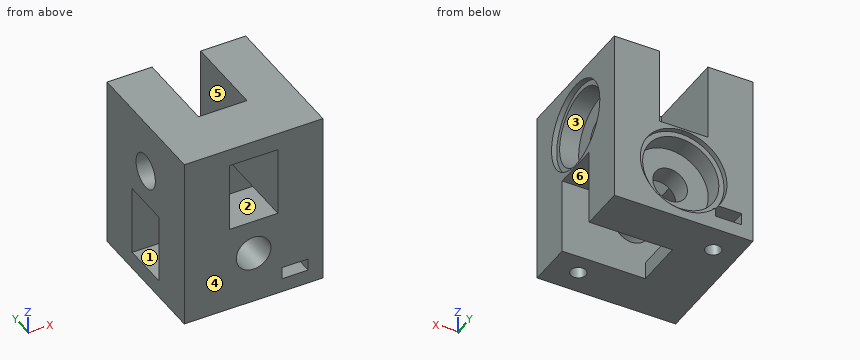
```python
from build123d import *

# Parameters (mm, degrees)
ESQUISSE1_W              = 40
ESQUISSE1_H              = 40
BOSS_EXTRU_1_DEPTH       = 50
ESQUISSE2_R              = 5
ENL_V_MAT_EXTRU_1_DEPTH  = 41
ESQUISSE3_R              = 5
ENL_V_MAT_EXTRU_2_DEPTH  = 41
ESQUISSE4_W              = 20
ESQUISSE4_H              = 14
ENL_V_MAT_EXTRU_3_DEPTH  = 29
ESQUISSE5_W              = 14
ESQUISSE5_H              = 20
ENL_V_MAT_EXTRU_4_DEPTH  = 29
ESQUISSE6_W              = 22
ESQUISSE6_H              = 14
ENL_V_MAT_EXTRU_5_DEPTH  = 24
ESQUISSE7_W              = 14
ESQUISSE7_H              = 22
ENL_V_MAT_EXTRU_6_DEPTH  = 24
ESQUISSE8_R              = 11
ENL_V_MAT_EXTRU_7_DEPTH  = 7
ESQUISSE9_R              = 12.5
ENL_V_MAT_EXTRU_8_DEPTH  = 1.5
ESQUISSE10_R             = 11
ENL_V_MAT_EXTRU_9_DEPTH  = 7
ESQUISSE11_R             = 12.5
ENL_V_MAT_EXTRU_10_DEPTH = 1.5
ESQUISSE13_R             = 2.2
ENL_V_MAT_EXTRU_11_DEPTH = 10
ESQUISSE15_W             = 7.5
ESQUISSE15_H             = 3.5
ENL_V_MAT_EXTRU_13_DEPTH = 12
ESQUISSE16_W             = 7.5
ESQUISSE16_H             = 3.5
ENL_V_MAT_EXTRU_14_DEPTH = 12


with BuildPart() as part:
    # Esquisse1 → Boss.-Extru.1 (new body)
    with BuildSketch(Plane.XY):
        with Locations((-20, 20)):
            Rectangle(ESQUISSE1_W, ESQUISSE1_H)
    extrude(amount=BOSS_EXTRU_1_DEPTH)

    # Esquisse2 → Enlèv. mat.-Extru.1 (cut, through all)
    with BuildSketch(Plane(origin=(0, 40, 0), x_dir=(1, 0, 0), z_dir=(0, 1, 0))):
        with Locations(Location((-20, -15, 0), (0, 0, 270))):  # turned: the seam where the file's is
            Circle(ESQUISSE2_R)
    extrude(amount=-ENL_V_MAT_EXTRU_1_DEPTH, mode=Mode.SUBTRACT)

    # Esquisse3 → Enlèv. mat.-Extru.2 (cut, through all)
    with BuildSketch(Plane.ZY.offset(40)):
        with Locations((35, 20)):
            Circle(ESQUISSE3_R)
    extrude(amount=-ENL_V_MAT_EXTRU_2_DEPTH, mode=Mode.SUBTRACT)

    # Esquisse4 → Enlèv. mat.-Extru.3 (cut)
    with BuildSketch(Plane.ZY.offset(40)):
        with Locations((15, 20)):
            Rectangle(ESQUISSE4_W, ESQUISSE4_H)
    extrude(amount=-ENL_V_MAT_EXTRU_3_DEPTH, mode=Mode.SUBTRACT)

    # Esquisse5 → Enlèv. mat.-Extru.4 (cut)
    with BuildSketch(Plane.XZ):
        with Locations((-20, 35)):
            Rectangle(ESQUISSE5_W, ESQUISSE5_H)
    extrude(amount=-ENL_V_MAT_EXTRU_4_DEPTH, mode=Mode.SUBTRACT)

    # Esquisse6 → Enlèv. mat.-Extru.5 (cut)
    with BuildSketch(Plane(origin=(0, 0, 0), x_dir=(0, 0, -1), z_dir=(1, 0, 0))):
        with Locations((-11, 20)):
            Rectangle(ESQUISSE6_W, ESQUISSE6_H)
    extrude(amount=-ENL_V_MAT_EXTRU_5_DEPTH, mode=Mode.SUBTRACT)

    # Esquisse7 → Enlèv. mat.-Extru.6 (cut)
    with BuildSketch(Plane(origin=(0, 40, 0), x_dir=(1, 0, 0), z_dir=(0, 1, 0))):
        with Locations((-20, -39)):
            Rectangle(ESQUISSE7_W, ESQUISSE7_H)
    extrude(amount=-ENL_V_MAT_EXTRU_6_DEPTH, mode=Mode.SUBTRACT)

    # Esquisse8 → Enlèv. mat.-Extru.7 (cut)
    with BuildSketch(Plane(origin=(0, 0, 0), x_dir=(0, 0, -1), z_dir=(1, 0, 0))):
        with Locations(Location((-35, 20, 0), (0, 0, 90))):  # turned: the seam where the file's is
            Circle(ESQUISSE8_R)
    extrude(amount=-ENL_V_MAT_EXTRU_7_DEPTH, mode=Mode.SUBTRACT)

    # Esquisse9 → Enlèv. mat.-Extru.8 (cut)
    with BuildSketch(Plane(origin=(0, 0, 0), x_dir=(0, 0, -1), z_dir=(1, 0, 0))):
        with Locations(Location((-35, 20, 0), (0, 0, 90))):  # turned: the seam where the file's is
            Circle(ESQUISSE9_R)
    extrude(amount=-ENL_V_MAT_EXTRU_8_DEPTH, mode=Mode.SUBTRACT)

    # Esquisse10 → Enlèv. mat.-Extru.9 (cut)
    with BuildSketch(Plane(origin=(0, 40, 0), x_dir=(1, 0, 0), z_dir=(0, 1, 0))):
        with Locations(Location((-20, -15, 0), (0, 0, 270))):  # turned: the seam where the file's is
            Circle(ESQUISSE10_R)
    extrude(amount=-ENL_V_MAT_EXTRU_9_DEPTH, mode=Mode.SUBTRACT)

    # Esquisse11 → Enlèv. mat.-Extru.10 (cut)
    with BuildSketch(Plane(origin=(0, 40, 0), x_dir=(1, 0, 0), z_dir=(0, 1, 0))):
        with Locations(Location((-20, -15, 0), (0, 0, 270))):  # turned: the seam where the file's is
            Circle(ESQUISSE11_R)
    extrude(amount=-ENL_V_MAT_EXTRU_10_DEPTH, mode=Mode.SUBTRACT)

    # Esquisse13 → Enlèv. mat.-Extru.11 (cut)
    with BuildSketch(Plane(origin=(0, 0, 0), x_dir=(-1, 0, 0), z_dir=(0, 0, -1))):
        with Locations((33, 32)):
            Circle(ESQUISSE13_R)
        with Locations((8, 7)):
            Circle(ESQUISSE13_R)
    extrude(amount=-ENL_V_MAT_EXTRU_11_DEPTH, mode=Mode.SUBTRACT)

    # Esquisse15 → Enlèv. mat.-Extru.13 (cut)
    with BuildSketch(Plane(origin=(0, 40, 0), x_dir=(1, 0, 0), z_dir=(0, 1, 0))):
        with Locations((-33, -5.75)):
            Rectangle(ESQUISSE15_W, ESQUISSE15_H)
    extrude(amount=-ENL_V_MAT_EXTRU_13_DEPTH, mode=Mode.SUBTRACT)

    # Esquisse16 → Enlèv. mat.-Extru.14 (cut)
    with BuildSketch(Plane.XZ):
        with Locations((-8, 5.75)):
            Rectangle(ESQUISSE16_W, ESQUISSE16_H)
    extrude(amount=-ENL_V_MAT_EXTRU_14_DEPTH, mode=Mode.SUBTRACT)


solid = part.part
```
For this review, take the finished solid that the model builds, in its own axes (mm). Face numbers are marked on the shaded views. A direction names the side the tool comes from. Coordinates: 2 decimals unless noted, no trailing zeros. Loops run counter-clockwise (first coordinate to the right, second up) from the corner with the lowest first, then second, coordinate; pieces in that order, holes last. Notation, with made-up numbers: (81, 18.5) -> (103, 18.5) arc R15 cw to (103, 22.5) -> close; hole circle Ø7 at (5.5, 37). An arc over 180 degrees is marked (long way). Return JSON: item names as keys, results as strings. Group by question number.
(1) Tool access review of the marked faces 1, 2 and 3: name each direction out of +Z, -Z, +X, -X, +Y, -Y from which nothing blocks a thin tool from reaching the whole face with its end or side.
(2) Mouldability with a two-part tool opening along Y and no side actions: class the marked faces 4, 5 and 6 as pulls with the +Y half, pulls with the -Y half, needs draft (parallel to the pull), parting line crosses it, or undercut.
(3) Consider section A-A, the plane y = 20. Count the separate pieces of the cut face and the enclosed holes in it, plus the area to 4 significant figures.
(4) Consider section C-C, the plane x = -26. Give the boundary of the cut face in (y, z), plus the area to 3 significant figures.
(5) For pin 1 Ø3.5 at (x, y) = (-7.5, 16.5) entering from -Z; pin 2 Ø5 at (y, z) = (20, 27.5) entering from +X; pin 3 Ø4 at (x, y) = (-17.5, 26.5) entering from +Z; pin 4 Ø2 at (y, z) = (24.5, 7.5) entering from -X, all flat-tipped, find the tip position at first contact; note any pin that passes through.
(6) Consider section B-B, the plane z = 35. Give the boundary of the cut face in (x, y), plus the area to 4 significant figures.
(7) To check wall thickness, follow L1, parallel to Z at x = -14, y = 2; L2, parallel to X at y = 6, z = 15; L3, parallel to Z at x = -32.5, y = 20. State the ranges of each line that lie inside material, in increasing order.
Results below:
{
 "1": {"face 1": "+X, -X", "face 2": "-Y", "face 3": "+X"},
 "2": {"face 4": "pulls with the -Y half", "face 5": "needs draft", "face 6": "undercut"},
 "3": {"separate pieces": "5", "enclosed holes": "0", "area": "414.5 mm2"},
 "4": {"outline": "(0, 0) -> (40, 0) -> (40, 4.03) -> (38.5, 4.03) -> (38.5, 5.78) -> (33, 5.78) -> (33, 24.22) -> (38.5, 24.22) -> (38.5, 25.97) -> (40, 25.97) -> (40, 28) -> (29, 28) -> (29, 25) -> (27, 25) -> (27, 5) -> (13, 5) -> (13, 25) -> (0, 25) -> close; (0, 45) -> (16, 45) -> (16, 50) -> (0, 50) -> close", "area": "699 mm2"},
 "5": {"pin 1": "stops at z = 22", "pin 2": "stops at x = -7", "pin 3": "stops at z = 25", "pin 4": "passes through"},
 "6": {"outline": "(-40, 0) -> (-27, 0) -> (-27, 15) -> (-40, 15) -> close; (-40, 25) -> (-27, 25) -> (-27, 40) -> (-40, 40) -> close; (-13, 0) -> (0, 0) -> (0, 7.5) -> (-1.5, 7.5) -> (-1.5, 9) -> (-7, 9) -> (-7, 15) -> (-13, 15) -> close; (-13, 25) -> (-7, 25) -> (-7, 31) -> (-1.5, 31) -> (-1.5, 32.5) -> (0, 32.5) -> (0, 40) -> (-13, 40) -> close", "area": "691.5 mm2"},
 "7": {"L1": "z = 0 to 25, 45 to 50", "L2": "x = -40 to -25, -15 to 0", "L3": "z = 0 to 5, 25 to 30, 40 to 50"}
}
